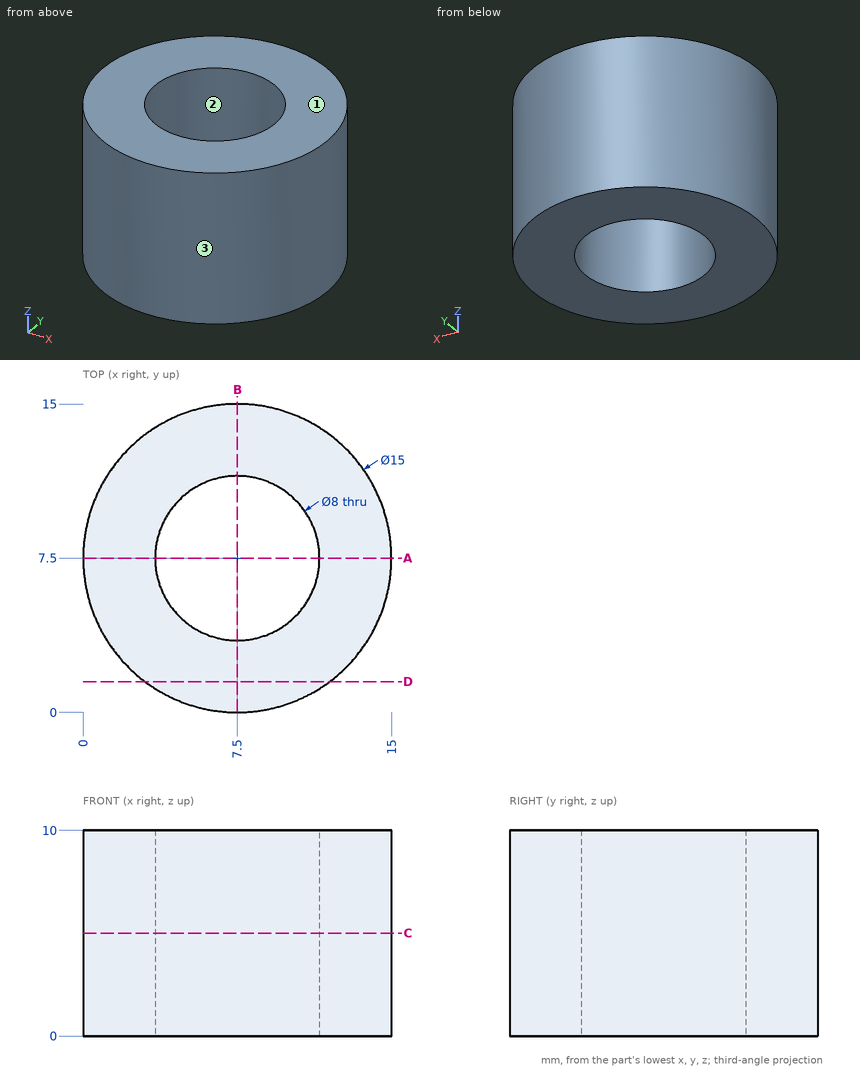
The figure shows three views and two pictorial views of one solid part (mm, origin at its lowest corner). Answer the questions. Give positions to 0.01 mm unless a question says otherwise; leave off trailing zeros. Loops run counter-clockwise (first coordinate to the right, second up) from the corner with the lowest first, then second, coordinate; pieces in that order, holes last. Notation, with made-up numbers: (46, -29) - (76, -29) arc R27 ccw to (76, -5) - close; hole circle Ø11 at (89.25, 49). An arc over 180 degrees is marked (long way). Use one line per item in the form item = value.
1. Section C-C on z = 5 is taken. Give the vertices of the cut face in (x, y), then the cut area to 3 significant figures.
Calculated:
outline = circle Ø15 at (7.5, 7.5); hole circle Ø8 at (7.5, 7.5)
area = 126 mm^2
2. The mould has two halves that part along X. Classify the marked faces 1, 2 and 3: pulls with the +X half, pulls with the -X half, needs draft (parallel to the pull), parting line crosses it, or undercut.
Calculated:
face_1 = needs draft
face_2 = undercut
face_3 = parting line crosses it
3. Section A-A on y = 7.5 is taken. Give the vertices of the cut face in (x, z).
Calculated:
outline = (0, 0) - (3.5, 0) - (3.5, 10) - (0, 10) - close; (11.5, 0) - (15, 0) - (15, 10) - (11.5, 10) - close
4. Given pin 1 Ø3 at (x, z) = (5, 3.5) entering from +Y; pin 2 Ø6 at (x, z) = (3, 6.5) entering from -Y; pin 3 Ø1.5 at (x, y) = (9, 4.5) entering from -Z; pin 4 Ø3 at (y, z) = (2.5, 8.5) entering from +X, each flat-ended and moving along its own axis, determine where each tip first touches the part or whether it passes through.
Calculated:
pin_1 = 14.93
pin_2 = 0.15
pin_3 = 0
pin_4 = 14.13
5. Find the intervals of material crossed by line 1 along Y through (x, z) = (7.5, 8.25); line 2 along X through (y, z) = (5.5, 7); line 3 along X through (y, z) = (5.75, 7), in increasing order. Write a range as [from, to].
Calculated:
line_1 = [0, 3.5], [11.5, 15]
line_2 = [0.27, 4.04], [10.96, 14.73]
line_3 = [0.21, 3.9], [11.1, 14.79]
6. Section D-D on y = 1.5 is taken. Give the vertices of the cut face in (x, z), then the cut area to 3 significant figures.
Calculated:
outline = (3, 0) - (12, 0) - (12, 10) - (3, 10) - close
area = 90.0 mm^2
